Verification items for the finished model (mm, model axes). Coordinates: 2 decimals unless noted, no trailing zeros. Loops run counter-clockwise (first coordinate to the right, second up) from the corner with the lowest first, then second, coordinate; pieces in that order, holes last. Notation, with made-up numbers: (80, 55) - (125, 55) arc R26 cw to (125, 89) - close; hole circle Ø1 at (0.5, 50). An arc over 180 degrees is marked (long way). Answer as CSV lines item,"result". Start each with the question number.
1. Cross-section at C-C (x = 56). Enter the section's corners in (y, z) (3 decimals).
2. Gauge pin test, flat ends, axial feed: P1, Ø1, axis at y = 1, z = 5, coming from the -X side; P2, Ø1.9, axis at x = 271, y = 1.5, coming from the +Z side (3 decimals); P3, Ø3, axis at y = -2.5, z = 4.5, coming from the +X side. Record the tip position at first contact, or that the pin passes through.
3. Material ranges on line 1 (X direction, y = -1, z = 4.25); line 2 (X direction, y = -0.25, z = 3.25); line 3 (Z direction, x = 352, y = 0.25) (3 decimals), recorded low to high. Write a range as [from, to].
4. Cross-section at A-A (z = 5). State how many separate pieces and enclosed holes the cut face has, plus the area to 3 significant figures.
5. Cross-section at B-B (y = -2). Enter the section's corners in (x, z) (3 decimals).
Autodesk Inventor part; units mm, degrees
ref_plane "YZ Plane" through (0, 0, 0) normal (1, 0, 0) x (0, 1, 0)
ref_plane "XZ Plane" through (0, 0, 0) normal (0, 1, 0) x (-1, 0, 0)
ref_plane "XY Plane" through (0, 0, 0) normal (0, 0, 1) x (1, 0, 0)
sketch "Sketch1" plane through (0, 0, 0) normal (0, 0, 1) x (1, 0, 0)
  line L0 (-44.3649, 2.907) -> (399.3477, 2.907)
  line L1 (399.3477, 2.907) -> (399.3477, -3.443)
  line L2 (399.3477, -3.443) -> (-44.3649, -3.443)
  line L3 (-44.3649, -3.443) -> (-44.3649, 2.907)
  point P0 (0, 0)
  dimension "d0" = 443.7126
  dimension "d1" = 6.35
extrude "Extrusion1" add sketch "Sketch1" along normal blind 3.175
sketch "Sketch2" plane through (0, 0, 3.175) normal (0, 0, 1) x (1, 0, 0)
  line L0 (399.3477, 2.907) -> (399.3477, -3.443)
  line L1 (-44.3649, 2.907) -> (399.3477, 2.907)
  line L2 (-44.3649, -3.443) -> (-44.3649, 2.907)
  line L3 (-44.3649, 2.907) -> (-44.3649, -0.268)
  line L4 (-44.3649, -0.268) -> (399.3477, -0.268)
  line L5 (399.3477, -0.268) -> (309.6603, -0.268)
  line L6 (-44.3649, -0.268) -> (45.3225, -0.268)
  circle A0 centre (-44.3649, -0.268) radius 3.175
  circle A1 centre (45.3225, -0.268) radius 3.175
  circle A2 centre (309.6603, -0.268) radius 3.175
  circle A3 centre (399.3477, -0.268) radius 3.175
  point P0 (0, 0)
  dimension "d4" = 3.175
  dimension "d5" = 89.6874
  dimension "d6" = 89.6874
extrude "Extrusion2" add sketch "Sketch2" along normal blind 3.175 contours A3 L0 | L0 L4 A3 | L0 A3 L4 | A2 L4 | A1 L4 | A2 L4 | A0 L4 L2 | L2 A0 | A1 L4 | L4 A0 L2
sketch "Sketch3" plane through (0, 0, 3.175) normal (0, 0, -1) x (-1, 0, 0)
  line L0 (-399.3477, 2.907) -> (-399.3477, -3.443)
  arc A0 (-399.3477, 2.907) -> (-399.3477, -3.443) centre (-399.3477, -0.268) ccw
  point P0 (0, 0)
extrude "Extrusion3" add sketch "Sketch3" along normal blind 3.175
sketch "Sketch4" plane through (0, 0, 3.175) normal (0, 0, -1) x (-1, 0, 0)
  line L0 (44.3649, -3.443) -> (44.3649, 2.907)
  arc A0 (44.3649, -3.443) -> (44.3649, 2.907) centre (44.3649, -0.268) ccw
  point P0 (0, 0)
extrude "Extrusion4" add sketch "Sketch4" along normal blind 3.175
sketch "Sketch5" plane through (0, 0, 3.175) normal (0, 0, 1) x (1, 0, 0)
  arc A0 (45.3225, -3.443) -> (45.3225, 2.907) centre (45.3225, -0.268) ccw
  line L0 (309.6603, -3.443) -> (45.3225, -3.443)
  arc A1 (309.6603, 2.907) -> (309.6603, -3.443) centre (309.6603, -0.268) ccw
  line L1 (45.3225, 2.907) -> (309.6603, 2.907)
  line L2 (309.6603, -3.443) -> (45.3225, 2.907)
  line L3 (45.3225, -3.443) -> (309.6603, 2.907)
  line L4 (177.4914, -0.268) -> (177.4914, -3.443)
  line L5 (181.9749, -3.443) -> (194.6749, -3.443)
  line L6 (194.6749, -3.443) -> (169.2749, -3.443)
  line L7 (169.2749, -3.443) -> (169.2749, 2.907)
  line L8 (169.2749, 2.907) -> (194.6749, 2.907)
  line L9 (194.6749, 2.907) -> (194.6749, -3.443)
  point P0 (0, 0)
  dimension "d13" = 12.7
  dimension "d14" = 25.4
extrude "Extrusion5" add sketch "Sketch5" along normal blind 3.175 contours L7 L3 L4 L0 | L7 L2 L3 | L1 L9 L3 L2 L7 | L4 L2 L9 L0 | L3 L9 L2
properties part number "connection"
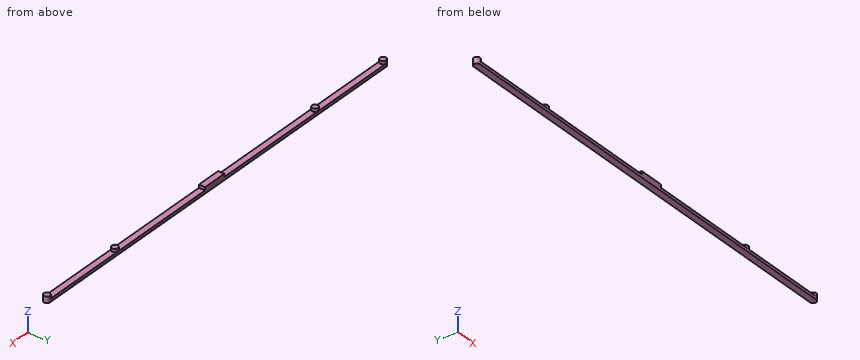
Values follow:
1,outline,"(-3.443, 0) - (2.907, 0) - (2.907, 3.175) - (-3.443, 3.175) - close"
2,P1,"stops at x = -47.45"
2,P2,"stops at z = 3.175"
2,P3,"stops at x = 402.44"
3,line 1,"x = [-47.45, -41.28], [42.23, 48.41], [169.27, 194.67], [306.57, 312.75], [396.26, 402.44]"
3,line 2,"x = [-47.54, -41.19], [42.15, 48.5], [169.27, 194.67], [306.49, 312.84], [396.17, 402.52]"
3,line 3,"z = [0, 3.175]"
4,separate pieces,"5"
4,enclosed holes,"0"
4,area,"288 mm²"
5,outline,"(-47.026, 0) - (402.009, 0) - (402.009, 6.35) - (396.687, 6.35) - (396.687, 3.175) - (312.321, 3.175) - (312.321, 6.35) - (306.999, 6.35) - (306.999, 3.175) - (194.675, 3.175) - (194.675, 6.35) - (169.275, 6.35) - (169.275, 3.175) - (47.983, 3.175) - (47.983, 6.35) - (42.662, 6.35) - (42.662, 3.175) - (-41.704, 3.175) - (-41.704, 6.35) - (-47.026, 6.35) - close"
